Work out the finished part from the listing and answer in its coordinate system (mm). A direction names the side the tool comes from. Round coordinates to 2 decimals unless told otherwise and drop trailing zeros. Loops run counter-clockwise (first coordinate to the right, second up) from the corner with the lowest first, then second, coordinate; pieces in that order, holes last.
from build123d import *
from build123d.topology import SkipClean

# Parameters (mm, degrees)
SKETCH2_R                 = 4.955
BOTTOM_OF_MOUNT_DEPTH     = 69.85
SKETCH3_R                 = 2.975
TOP_OF_MOUNT_DEPTH        = 6.35
SKETCH4_R                 = 1
SCREW_CUT_IN_BOTTOM_DEPTH = 20
LOCK_IN_HOLE_DEPTH        = 77.52152671
LOCK_IN_HOLE_DEPTH_BACK   = 77.52152671
SKETCH6_R                 = 0.9
FILLET5_R                 = 0.5


with BuildPart() as part:
    # Sketch2 → Bottom of Mount (new body)
    with BuildSketch(Plane(origin=(0, 0, 0), x_dir=(1, 0, 0), z_dir=(0, 1, 0))):
        with Locations(Location((0, 0, 0), (0, 0, 270))):
            Circle(SKETCH2_R)
    extrude(amount=BOTTOM_OF_MOUNT_DEPTH)

    # Sketch3 → Top of Mount (add)
    with BuildSketch(Plane(origin=(0, 69.85, 0), x_dir=(1, 0, 0), z_dir=(0, 1, 0))):
        with Locations(Location((0, 0, 0), (0, 0, 270))):
            Circle(SKETCH3_R)
    extrude(amount=TOP_OF_MOUNT_DEPTH)

    # Sketch4 → Screw Cut in Bottom (cut)
    with BuildSketch(Plane.XZ):
        with Locations(Location((0, 0, 0), (0, 0, 270))):
            Circle(SKETCH4_R)
    extrude(amount=-SCREW_CUT_IN_BOTTOM_DEPTH, mode=Mode.SUBTRACT)

    # Sketch6 → Lock in hole (cut, two sides: drawn at the far end of the back side and taken through both)
    with BuildSketch(Plane.XY.offset(-LOCK_IN_HOLE_DEPTH_BACK)):
        with Locations(Location((0, 73.39, 0), (0, 0, 89.999999984))):
            Circle(SKETCH6_R)
    extrude(amount=LOCK_IN_HOLE_DEPTH + LOCK_IN_HOLE_DEPTH_BACK, mode=Mode.SUBTRACT)

    # Sketch9 → Circular Top (revolve)
    with SkipClean():  # the faces are left unmerged after this step: merging them gives an invalid solid
        with BuildSketch(Plane.XY):
            with BuildLine():
                Line((2.975, 76.2), (-2.975, 76.2))
                ThreePointArc((-2.975, 76.2), (0, 79.175), (2.975, 76.2))
            make_face()
        revolve(axis=Axis((2.975, 76.2, 0), (-1, 0, 0)))

    # Fillet5
    fillet5_edges = [part.edges().sort_by_distance(p)[0] for p in [
        (0, 69.85, -4.955),
    ]]
    fillet(fillet5_edges, radius=FILLET5_R)


solid = part.part
Item 1: For faces 4 (the face through (-1, 10, 0)), 5 (the face through (1.488, 34.19, 4.726)), determine the directions among +Z, -Z, +X, -X, +Y, -Y from which every point of the face is accessible in a straight line to the end or side of a thin tool.
Item 2: Each of these flat-tipped pins is pushed along its axis until it touches: P1, Ø1.4, axis at x = 0, y = 73.39, coming from the +Z side; P2, Ø5, axis at x = -4, z = 1, coming from the +Y side; P3, Ø3, axis at x = -1.5, z = 3.5, coming from the +Y side. Where does it stop, or does it pass through?
Item 3: Straight lines are drawn through the part: line 1 (X direction, y = 5.5, z = 0) (3 decimals); line 2 (Y direction, x = 0, z = 0.15); line 3 (Y direction, x = 0, z = -1.6). For each, find the intervals that lie inside material, in ascending order.
Item 4: Section A-A, the plane x = 0 is taken. Give the vertices of the cut face in (y, z) (3 decimals).
Item 5: Section B-B, the plane z = 0 is taken. Give the vertices of the cut face in (x, y) (3 decimals), plus the area to 3 significant figures.
Item 6: Section C-C, the plane y = 27 is taken. Give the vertices of the cut face in (x, z) (3 decimals), plus the area to 3 significant figures.
Item 7: Determine the mould class of faces 1 (the face through (0, 20, 0)), 2 (the face through (-1.14, 72.98, 2.75)), 3 (the face through (-3, 69.85, 1)) for opening direction X: pulls with the +X half, pulls with the -X half, needs draft (parallel to the pull), parting line crosses it, or undercut.
Answer below:
1. face 4: -Y
1. face 5: +Y, -Y
2. P1: stops at z = 2.1
2. P2: stops at y = 78.69
2. P3: stops at y = 78.08
3. line 1: x = -4.955 to -1, 1 to 4.955
3. line 2: y = 20 to 72.49, 73.23 to 79.17
3. line 3: y = 0 to 72.49, 73.69 to 78.71
4. outline: (0, -4.955) - (69.35, -4.955) arc R0.5 ccw to (69.85, -4.455) - (69.85, -2.975) - (72.49, -2.975) - (72.49, 2.975) - (69.85, 2.975) - (69.85, 4.455) arc R0.5 ccw to (69.35, 4.955) - (0, 4.955) - (0, 1) - (20, 1) - (20, -1) - (0, -1) - close; (74.29, -2.975) - (76.2, -2.975) arc R2.975 ccw to (76.2, 2.975) - (74.29, 2.975) - (74.29, 2.281) arc R2.975 ccw to (74.29, -2.281) - close
5. outline: (-4.955, 0) - (-1, 0) - (-1, 20) - (1, 20) - (1, 0) - (4.955, 0) - (4.955, 69.35) arc R0.5 ccw to (4.455, 69.85) - (2.975, 69.85) - (2.975, 76.2) arc R2.975 ccw to (-2.975, 76.2) - (-2.975, 69.85) - (-4.455, 69.85) arc R0.5 ccw to (-4.955, 69.35) - close; hole (-0.9, 73.364) arc R0.9 ccw to (0.9, 73.364) arc R2.975 cw to start
5. area: 703 mm2
6. outline: circle Ø9.91 at (0, 0)
6. area: 77.1 mm2
7. face 1: undercut
7. face 2: parting line crosses it
7. face 3: needs draft
